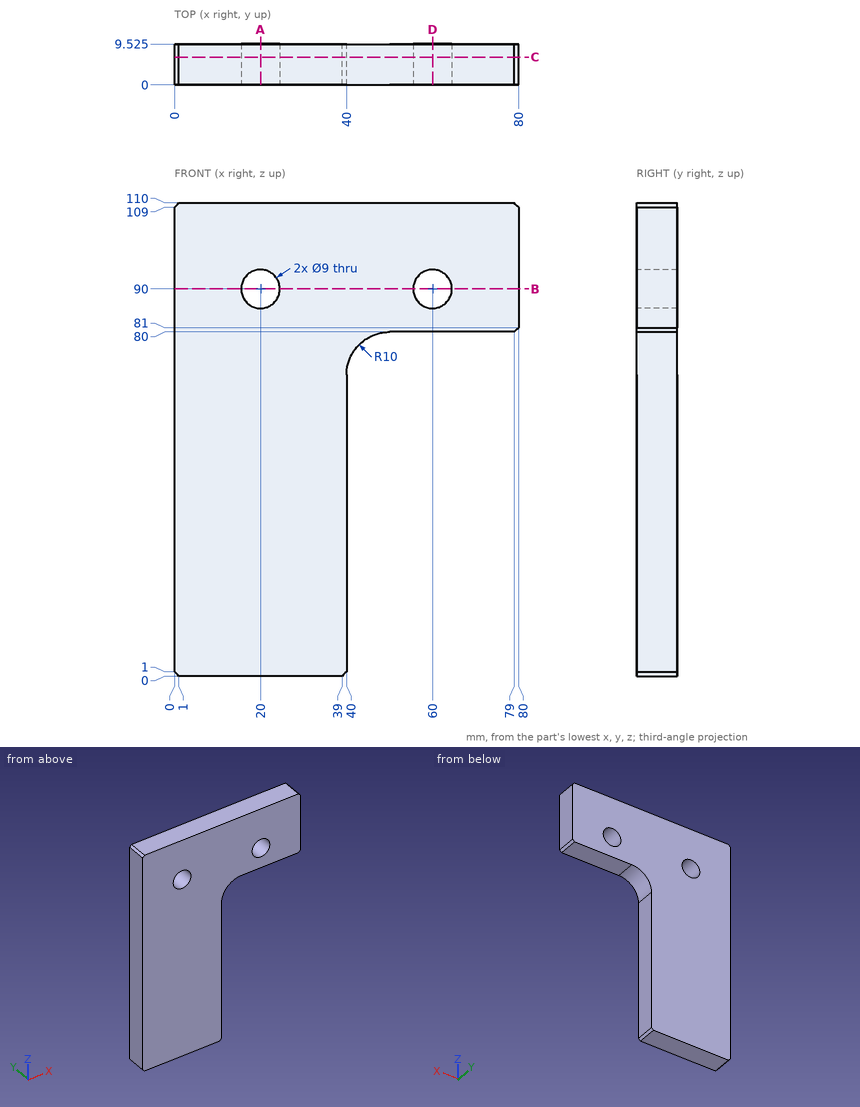
Answer from the drawing. Dimensions are ordinates in mm from the lowest x, y and z of the part. Round coordinates to 2 decimals unless told otherwise and drop trailing zeros. Write each loop counter-clockwise with the first axis right and the second up, starting at its lowest first coordinate (ties: lowest second). Pieces come first, ordered by that corner, then holes. Notation, with made-up numbers: M -14.5,33 L -10.5,33 A4 ccw -10.5,40 Z; hole C -14.5,-7 d9. An arc over 180 degrees is marked long. Write each question's results on one line, items separated by ' | '. Start each with the question number.
Item 1: Find section C-C on y = 6.5. Write down the section's boundary in (x, z).
Item 2: Find section B-B on z = 90. Write down the section's boundary in (x, y) (3 decimals), and give its area (3 significant figures).
Item 3: Straight lines are drawn through the part: probe 1 along X at (y, z) = (6.75, 90); probe 2 along Z at (x, y) = (60, 6); probe 3 along Z at (x, y) = (20, 4.75). For each, find the intervals that lie inside material, in ascending order.
Item 4: Find section A-A on x = 20. Write down the section's boundary in (y, z) (3 decimals).
Item 5: Given pin 1 Ø5 at (x, y) = (23, 5) entering from -Z; pin 2 Ø3 at (x, y) = (71.5, 7) entering from -Z; pin 3 Ø8 at (x, z) = (20, 90) entering from -Y; pin 4 Ø5 at (y, z) = (3, 52.5) entering from +X, each flat-ended and moving along its own axis, determine where each tip first touches the part or whether it passes through.
Item 6: Find section D-D on x = 60. Write down the section's boundary in (y, z) (3 decimals).
Answer block:
1) outline: M 0,1 L 1,0 L 39,0 L 40,1 L 40,70 A10 cw 50,80 L 79,80 L 80,81 L 80,109 L 79,110 L 1,110 L 0,109 Z; hole C 20,90 d9; hole C 60,90 d9
2) outline: M 0,0 L 15.5,0 L 15.5,9.525 L 0,9.525 Z; M 24.5,0 L 55.5,0 L 55.5,9.525 L 24.5,9.525 Z; M 64.5,0 L 80,0 L 80,9.525 L 64.5,9.525 Z | area: 591 mm²
3) probe 1: x = 0 to 15.5, 24.5 to 55.5, 64.5 to 80 | probe 2: z = 80 to 85.5, 94.5 to 110 | probe 3: z = 0 to 85.5, 94.5 to 110
4) outline: M 0,0 L 9.525,0 L 9.525,85.5 L 0,85.5 Z; M 0,94.5 L 9.525,94.5 L 9.525,110 L 0,110 Z
5) pin 1: stops at z = 0 | pin 2: stops at z = 80 | pin 3: passes through | pin 4: stops at x = 40
6) outline: M 0,80 L 9.525,80 L 9.525,85.5 L 0,85.5 Z; M 0,94.5 L 9.525,94.5 L 9.525,110 L 0,110 Z
